Check sheet for the modelled part. Datum: model origin and axes. Units: mm. A direction names the side the tool comes from. Give positions to 0.01 mm unless a question says otherwise; leave off trailing zeros. Loops run counter-clockwise (first coordinate to the right, second up) from the corner with the lowest first, then second, coordinate; pieces in that order, holes last. Notation, with made-up numbers: M 73,-0.75 L 114,-0.75 A20 ccw 114,3.25 Z; hole C -29.75,75.25 d5. An arc over 180 degrees is marked long. Write each question's results on one line, items separated by ' | '. Start each with the question number.
1. Material ranges on line 1 along Y through (x, z) = (386, 25); line 2 along X through (y, z) = (-25.5, -74.5); line 3 along Y through (x, z) = (459.5, -183.5), recorded low to high.
2. Sectioned sample at B-B on y = 25. Record the cut outline in (x, z).
3. Sectioned sample at D-D on x = 367. Record the cut outline in (y, z).
4. Go/stop test with flat-tipped pins: pin 1 (12 mm diameter, centred on x = 163, y = 34, fed in from +Z); pin 2 (6 mm diameter, centred on y = 32, z = -168, fed in from +X). Record where each tip stops, or that it passes through.
5. Tool access check on faces 1 (the flat face through (350, 1, -175)), 2 (the flat face through (400, 11, -77)), 3 (the flat face through (391, -12, 50)), 4 (the flat face through (202, 1, 0)). Record the directions out of +Z, -Z, +X, -X, +Y, -Y that give a thin tool (end or side, any length) a straight path to the whole face; none if there is none.
6. Sectioned sample at C-C on y = 3.5. Record the cut outline in (x, z), and give its area (3 significant figures).
7. Draft check along Y on faces 5 (the cylindrical face through (25.35, 21.17, -184.237)), 6 (the flat face through (449, -30, -73)), 7 (the flat face through (198, 1, -150)). Enter one of: pulls with the +Y half, pulls with the -Y half, needs draft (parallel to the pull), parting line crosses it, or undercut.
8. Sectioned sample at A-A on z = 25. Record the cut outline in (x, y).
```python
from build123d import *

# Parameters (mm, degrees)
SKETCH2_W           = 400
SKETCH2_H           = 150
BOSS_EXTRUDE1_DEPTH = 50
SKETCH3_W           = 50
SKETCH3_H           = 50
BOSS_EXTRUDE2_DEPTH = 50
SKETCH4_R           = 10
CUT_EXTRUDE1_DEPTH  = 444
BOSS_EXTRUDE3_DEPTH = 50
SKETCH7_W           = 250
SKETCH7_H           = 20
BOSS_EXTRUDE4_DEPTH = 100


with BuildPart() as part:
    # Sketch2 → Boss-Extrude1 (new body)
    with BuildSketch(Plane(origin=(0, 0, 0), x_dir=(1, 0, 0), z_dir=(0, 1, 0))):
        with Locations((200, 75)):
            Rectangle(SKETCH2_W, SKETCH2_H)
    extrude(amount=BOSS_EXTRUDE1_DEPTH)

    # Sketch3 → Boss-Extrude2 (add)
    with BuildSketch(Plane(origin=(400, 0, 0), x_dir=(0, 0, -1), z_dir=(1, 0, 0))):
        with Locations((-25, 25)):
            Rectangle(SKETCH3_W, SKETCH3_H)
        with Locations((175, 25)):
            Rectangle(SKETCH3_W, SKETCH3_H)
    boss_extrude2 = extrude(amount=-BOSS_EXTRUDE2_DEPTH)

    # Mirror4: Boss-Extrude2 across plane
    add(boss_extrude2.mirror(Plane(origin=(200, 0, 0), x_dir=(0, 0, 1), z_dir=(1, 0, 0))))

    # Sketch4 → Cut-Extrude1 (cut)
    with BuildSketch(Plane(origin=(400, 0, 0), x_dir=(0, 0, -1), z_dir=(1, 0, 0))):
        with Locations((-25, 25)):
            Circle(SKETCH4_R)
        with Locations((175, 25)):
            Circle(SKETCH4_R)
    extrude(amount=-CUT_EXTRUDE1_DEPTH, mode=Mode.SUBTRACT)

    # Sketch6 → Boss-Extrude3 (add)
    with BuildSketch(Plane.XZ):
        Polygon((0, 50), (0, -200), (50, -200), (50, -150), (350, -150), (350, -200), (400, -200), (400, 50), (350, 50), (350, 0), (50, 0), (50, 50), align=None)
    extrude(amount=BOSS_EXTRUDE3_DEPTH)

    # Sketch7 → Boss-Extrude4 (add)
    with BuildSketch(Plane(origin=(400, 0, 0), x_dir=(0, 0, -1), z_dir=(1, 0, 0))):
        with Locations((75, -40)):
            Rectangle(SKETCH7_W, SKETCH7_H)
    extrude(amount=BOSS_EXTRUDE4_DEPTH)


solid = part.part
```
Output values:
1) line 1: -50 to 15, 35 to 50 | line 2: 0 to 400 | line 3: -50 to -30
2) outline: M 0,-200 L 50,-200 L 50,-185 L 0,-185 Z; M 0,-165 L 50,-165 L 50,-150 L 350,-150 L 350,-165 L 400,-165 L 400,15 L 350,15 L 350,0 L 50,0 L 50,15 L 0,15 Z; M 0,35 L 50,35 L 50,50 L 0,50 Z; M 350,-200 L 400,-200 L 400,-185 L 350,-185 Z; M 350,35 L 400,35 L 400,50 L 350,50 Z
3) outline: M -50,-200 L 50,-200 L 50,50 L -50,50 Z; hole C 25,-175 d20; hole C 25,25 d20
4) pin 1: z = 0 | pin 2: x = 400
5) face 1: -Z, +Y, -Y | face 2: +Z, -Z, +X, +Y | face 3: +Z, +X, -X, +Y, -Y | face 4: +Z, +Y, -Y
6) outline: M 0,-200 L 50,-200 L 50,-150 L 350,-150 L 350,-200 L 400,-200 L 400,50 L 350,50 L 350,0 L 50,0 L 50,50 L 0,50 Z | area: 70,000 mm2
7) face 5: undercut | face 6: pulls with the +Y half | face 7: needs draft
8) outline: M 0,-50 L 50,-50 L 50,15 L 0,15 Z; M 0,35 L 50,35 L 50,50 L 0,50 Z; M 350,-50 L 500,-50 L 500,-30 L 400,-30 L 400,15 L 350,15 Z; M 350,35 L 400,35 L 400,50 L 350,50 Z
